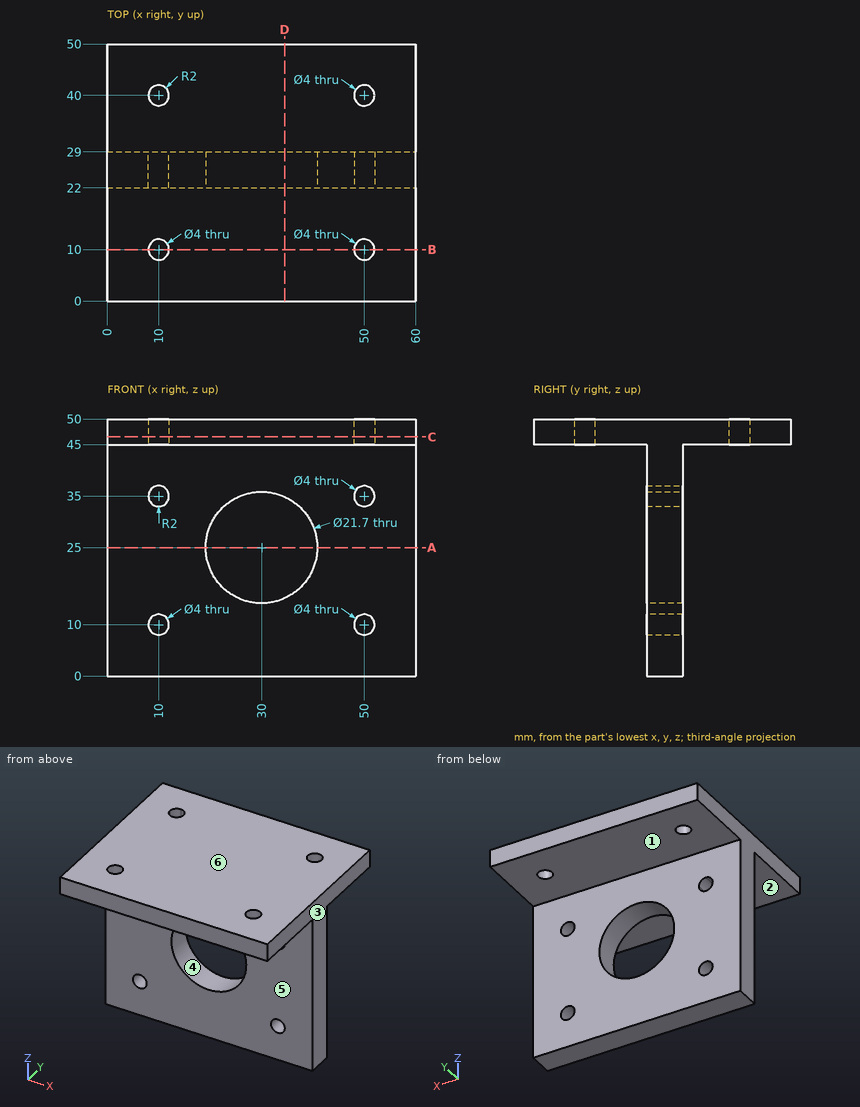
Could you check a few things on this drawing? It's one solid part, dimensions in mm from its lowest x, y, z. A direction names the side the tool comes from. Round coordinates to 2 decimals unless told otherwise and drop trailing zeros. Write each loop counter-clockwise with the first axis right and the second up, starting at its lowest first coordinate (ties: lowest second). Pieces come first, ordered by that corner, then holes. Notation, with made-up numbers: (-36.5, 50.25) -> (-28.5, 50.25) arc R28 cw to (-28.5, 83.25) -> close; hole circle Ø4 at (58, 26.25). An arc over 180 degrees is marked (long way). Use a Markdown table: item, result.
1. Please list where these lines run through material, in increasing order: probe 1 along X at (y, z) = (25, 10); probe 2 along Y at (x, z) = (21.5, 7); probe 3 along Z at (x, y) = (55.5, 6.5).
Answer key:
| item | result |
|---|---|
| probe 1 | x = 0 to 8, 12 to 48, 52 to 60 |
| probe 2 | y = 22 to 29 |
| probe 3 | z = 45 to 50 |
2. If we section it at A-A (z = 25): List the corners of the cut face in (x, y) for me.
Answer key:
| item | result |
|---|---|
| outline | (0, 22) -> (19.15, 22) -> (19.15, 29) -> (0, 29) -> close; (40.85, 22) -> (60, 22) -> (60, 29) -> (40.85, 29) -> close |
3. If we section it at C-C (z = 46.5): List the corners of the cut face in (x, y) for me.
Answer key:
| item | result |
|---|---|
| outline | (0, 0) -> (60, 0) -> (60, 50) -> (0, 50) -> close; hole circle Ø4 at (10, 10); hole circle Ø4 at (10, 40); hole circle Ø4 at (50, 10); hole circle Ø4 at (50, 40) |
4. If we section it at D-D (x = 34.5): List the corners of the cut face in (y, z) for me, then the cut area to 3 significant figures.
Answer key:
| item | result |
|---|---|
| outline | (0, 45) -> (22, 45) -> (22, 34.87) -> (29, 34.87) -> (29, 45) -> (50, 45) -> (50, 50) -> (0, 50) -> close; (22, 0) -> (29, 0) -> (29, 15.13) -> (22, 15.13) -> close |
| area | 427 mm^2 |
5. Which directions (+Z, -Z, +X, -X, +Y, -Y) give clear straight access to the entire face, cutting with the end or side of a thin tool? Please do the marked faces 1, 2 and 3.
Answer key:
| item | result |
|---|---|
| face 1 | -Z, +X, -X, +Y |
| face 2 | -Z, +X, -X, -Y |
| face 3 | +Z, -Z, +X, +Y, -Y |
6. We'd pull the mould along Z, two halves only. Please class the marked faces 4, 5 and 6: +Z half, -Z half, draft (parallel to the pull), parting line (faces both ways), or undercut.
Answer key:
| item | result |
|---|---|
| face 4 | undercut |
| face 5 | draft |
| face 6 | +Z half |
7. If we section it at B-B (y = 10): List the corners of the cut face in (x, z) for me, then the cut area to 3 significant figures.
Answer key:
| item | result |
|---|---|
| outline | (0, 45) -> (8, 45) -> (8, 50) -> (0, 50) -> close; (12, 45) -> (48, 45) -> (48, 50) -> (12, 50) -> close; (52, 45) -> (60, 45) -> (60, 50) -> (52, 50) -> close |
| area | 260 mm^2 |
8. For pin 1 Ø6.5 at (x, y) = (10, 10) entering from +Z; pin 2 Ø6 at (x, z) = (50.5, 26.5) entering from +Y; pin 3 Ø12 at (x, z) = (21.5, 34.5) entering from -Y; pin 4 Ø2.5 at (x, z) = (10, 10) entering from +Y, each with a flat end and sliding along its axis, tell me the tip position at first contact or that it passes through.
Answer key:
| item | result |
|---|---|
| pin 1 | stops at z = 50 |
| pin 2 | stops at y = 29 |
| pin 3 | stops at y = 22 |
| pin 4 | passes through |
